Work out the finished part from the listing and answer in its coordinate system (mm). Face numbers are marked on the shaded views. A direction names the side the tool comes from. Coordinates: 2 decimals unless noted, no trailing zeros. Loops run counter-clockwise (first coordinate to the right, second up) from the corner with the lowest first, then second, coordinate; pieces in that order, holes last. Notation, with made-up numbers: (-30.75, 63.25) - (-9.75, 63.25) arc R17 ccw to (-9.75, 69.25) - close; hole circle Ø3 at (76, 21). An arc over 180 degrees is marked (long way). Write each question's results on one line, items separated by ' | '. Start each with the question number.
1. Determine the mould class of the marked faces 1, 2, 3 and 4 for opening direction Z: released by +Z, released by -Z, zero draft, split by the parting line, or undercut.
2. Find the intervals of material crossed by line 1 along Z through (x, y) = (11, 10.25); line 2 along Z through (x, y) = (12, 6.5); line 3 along Y through (x, z) = (4.5, 6.25), in increasing order. Write a range as [from, to].
3. A cutting plane is placed at A-A on z = 2. Determine the outline of the cut face in (x, y).
4. A cutting plane is placed at C-C on y = 14. Determine the outline of the cut face in (x, z).
5. A cutting plane is placed at D-D on y = 4. Determine the outline of the cut face in (x, z).
6. Which of the six approach directions +Z, -Z, +X, -X, +Y, -Y give full straight-line access (tool end or side, diameter ignored) to the marked faces 5 and 6?
7. A cutting plane is placed at B-B on x = 4.5. Determine the outline of the cut face in (y, z).
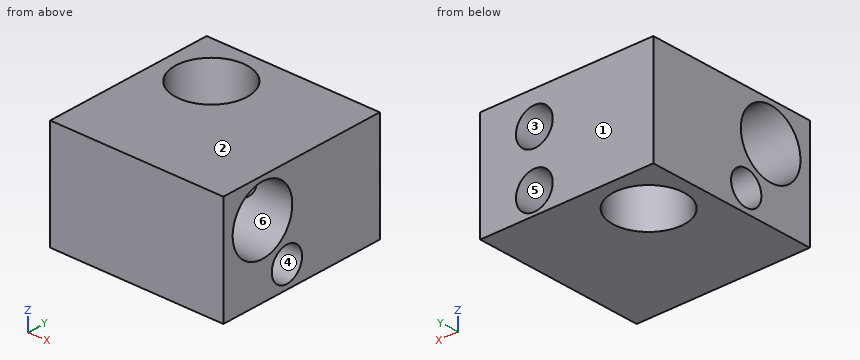
from build123d import *

# Parameters (mm, degrees)
ESQUISSE1_W                     = 16
ESQUISSE1_H                     = 16
BOSS_EXTRU_1_DEPTH              = 10
D_GAGEMENT_M61_D                = 6.6
DIAM_TRE_DU_PER_AGE_6_1_6_1_1_D = 6.1
DIAM_TRE_DU_PER_AGE_3_1_3_1_1_D = 3.1
D_GAGEMENT_M31_D                = 3.4
D_GAGEMENT_M31_DEPTH            = 11
D_GAGEMENT_M31_TIP              = 1.021463052
D_GAGEMENT_M33_D                = 3.4
D_GAGEMENT_M33_DEPTH            = 9.5
D_GAGEMENT_M33_TIP              = 1.021463052


with BuildPart() as part:
    # Esquisse1 → Boss.-Extru.1 (new body)
    with BuildSketch(Plane.XY):
        with Locations((8, 8)):
            Rectangle(ESQUISSE1_W, ESQUISSE1_H)
    extrude(amount=BOSS_EXTRU_1_DEPTH)

    # Dégagement M61 (through all)
    with Locations(Plane.XY.offset(10)):
        with Locations((4.5, 11.5)):
            Hole(D_GAGEMENT_M61_D / 2)

    # Diamètre du perçage Ø6.1 (6.1)1 (through all)
    with Locations(Plane(origin=(16, 0, 0), x_dir=(0, 0, -1), z_dir=(1, 0, 0))):
        with Locations((-6.5, 4)):
            Hole(DIAM_TRE_DU_PER_AGE_6_1_6_1_1_D / 2)

    # Diamètre du perçage Ø3.1 (3.1)1 (through all)
    with Locations(Plane(origin=(16, 0, 0), x_dir=(0, 0, -1), z_dir=(1, 0, 0))):
        with Locations((-2, 6.5)):
            Hole(DIAM_TRE_DU_PER_AGE_3_1_3_1_1_D / 2)

    # Dégagement M31
    with Locations(Plane(origin=(0, 16, 0), x_dir=(1, 0, 0), z_dir=(0, 1, 0))):
        with Locations((11, -7)):
            Hole(D_GAGEMENT_M31_D / 2, depth=D_GAGEMENT_M31_DEPTH)
            with Locations((0, 0, -(D_GAGEMENT_M31_DEPTH + D_GAGEMENT_M31_TIP / 2))):  # 118° drill point
                Cone(0, D_GAGEMENT_M31_D / 2, D_GAGEMENT_M31_TIP, mode=Mode.SUBTRACT)

    # Dégagement M33
    with Locations(Plane(origin=(0, 16, 0), x_dir=(1, 0, 0), z_dir=(0, 1, 0))):
        with Locations((11, -2)):
            Hole(D_GAGEMENT_M33_D / 2, depth=D_GAGEMENT_M33_DEPTH)
            with Locations((0, 0, -(D_GAGEMENT_M33_DEPTH + D_GAGEMENT_M33_TIP / 2))):  # 118° drill point
                Cone(0, D_GAGEMENT_M33_D / 2, D_GAGEMENT_M33_TIP, mode=Mode.SUBTRACT)


solid = part.part
Values:
1) face 1: zero draft | face 2: released by +Z | face 3: undercut | face 4: undercut
2) line 1: [0, 0.3], [3.7, 5.3], [8.7, 10] | line 2: [0, 0.45], [3.55, 4.75], [8.37, 10] | line 3: [0, 0.96], [7.04, 8.2], [14.8, 16]
3) outline: (0, 0) - (16, 0) - (16, 4.95) - (0, 4.95) - close; (0, 8.05) - (9.3, 8.05) - (9.3, 16) - (0, 16) - close; (12.7, 8.05) - (16, 8.05) - (16, 16) - (12.7, 16) - close; hole circle Ø6.6 at (4.5, 11.5)
4) outline: (0, 0) - (2.35, 0) - (2.35, 10) - (0, 10) - close; (6.65, 0) - (16, 0) - (16, 10) - (6.65, 10) - close; hole circle Ø3.4 at (11, 2); hole circle Ø3.4 at (11, 7)
5) outline: (0, 0) - (16, 0) - (16, 3.45) - (0, 3.45) - close; (0, 9.55) - (16, 9.55) - (16, 10) - (0, 10) - close
6) face 5: +Y | face 6: +X, -X
7) outline: (0, 0) - (8.2, 0) - (8.2, 10) - (0, 10) - close; (14.8, 0) - (16, 0) - (16, 10) - (14.8, 10) - close; hole circle Ø6.1 at (4, 6.5); hole circle Ø3.1 at (6.5, 2)
